```python
from build123d import *

# Parameters (mm, degrees)
CYLINDER959_R           = 1.6
CYLINDER959_DEPTH       = 10
CYLINDER959_PITCH_ANGLE = 90
CYLINDER960_R           = 1.6
CYLINDER960_DEPTH       = 10
CYLINDER960_PITCH_ANGLE = 90
CYLINDER962_R           = 3.1
CYLINDER962_DEPTH       = 2.5
CYLINDER962_PITCH_ANGLE = 90
CYLINDER961_R           = 3.1
CYLINDER961_DEPTH       = 2.5
CYLINDER961_PITCH_ANGLE = 90
BOX562_W                = 41
BOX562_H                = 41
BOX562_DEPTH            = 26
CYLINDER958_R           = 6
CYLINDER958_DEPTH       = 11
CYLINDER958_ROLL_ANGLE  = 90
CYLINDER963_R           = 7
CYLINDER963_DEPTH       = 5
CYLINDER963_ROLL_ANGLE  = 90
BOX563_W                = 10
BOX563_H                = 10
BOX563_DEPTH            = 17
CYLINDER953_R           = 1.2
CYLINDER953_DEPTH       = 10
CYLINDER953_ROLL_ANGLE  = 90
CYLINDER952_R           = 1.2
CYLINDER952_DEPTH       = 10
CYLINDER952_ROLL_ANGLE  = 90
CYLINDER957_R           = 1.25
CYLINDER957_DEPTH       = 15
CYLINDER957_PITCH_ANGLE = 90
CYLINDER955_R           = 1.25
CYLINDER955_DEPTH       = 11
CYLINDER955_PITCH_ANGLE = 90
CYLINDER956_R           = 1.25
CYLINDER956_DEPTH       = 15
CYLINDER956_PITCH_ANGLE = 90
CYLINDER954_R           = 1.25
CYLINDER954_DEPTH       = 11
CYLINDER954_PITCH_ANGLE = 90
BOX561_W                = 10
BOX561_H                = 63
BOX561_DEPTH            = 25.5
FILLET358_R             = 3
BOX560_W                = 16
BOX560_H                = 60
BOX560_DEPTH            = 17
FILLET359_R             = 3


with BuildPart() as cylinder1122:
    # Cylinder959 → Cylinder959 (new body)
    with BuildSketch(Plane.XY):
        Circle(CYLINDER959_R)
    extrude(amount=CYLINDER959_DEPTH)


with BuildPart() as cylinder1122_1:
    # Cylinder959 pitch: moved
    add(cylinder1122.part.rotate(Axis((0, 0, 0), (0, 1, 0)), CYLINDER959_PITCH_ANGLE))


with BuildPart() as cylinder1122_2:
    # Cylinder959 placement: moved
    add(cylinder1122_1.part.moved(Location((13.5, 83, -11))))


with BuildPart() as cylinder1123:
    # Cylinder960 → Cylinder960 (new body)
    with BuildSketch(Plane.XY):
        Circle(CYLINDER960_R)
    extrude(amount=CYLINDER960_DEPTH)


with BuildPart() as cylinder1123_1:
    # Cylinder960 pitch: moved
    add(cylinder1123.part.rotate(Axis((0, 0, 0), (0, 1, 0)), CYLINDER960_PITCH_ANGLE))


with BuildPart() as cylinder1123_2:
    # Cylinder960 placement: moved
    add(cylinder1123_1.part.moved(Location((13.5, 91, -11))))


with BuildPart() as cylinder1125:
    # Cylinder962 → Cylinder962 (new body)
    with BuildSketch(Plane.XY):
        Circle(CYLINDER962_R)
    extrude(amount=CYLINDER962_DEPTH)


with BuildPart() as cylinder1125_1:
    # Cylinder962 pitch: moved
    add(cylinder1125.part.rotate(Axis((0, 0, 0), (0, 1, 0)), CYLINDER962_PITCH_ANGLE))


with BuildPart() as cylinder1125_2:
    # Cylinder962 placement: moved
    add(cylinder1125_1.part.moved(Location((13.5, 83, -11))))


with BuildPart() as fusion603:
    # Cylinder961 → Cylinder961 (new body)
    with BuildSketch(Plane.XY):
        Circle(CYLINDER961_R)
    extrude(amount=CYLINDER961_DEPTH)


with BuildPart() as fusion603_1:
    # Cylinder961 pitch: moved
    add(fusion603.part.rotate(Axis((0, 0, 0), (0, 1, 0)), CYLINDER961_PITCH_ANGLE))


with BuildPart() as fusion603_2:
    # Cylinder961 placement: moved
    add(fusion603_1.part.moved(Location((13.5, 91, -11))))

    # Fusion603: union Cylinder1122, Cylinder1123, Cylinder1125
    add(cylinder1122_2.part)
    add(cylinder1123_2.part)
    add(cylinder1125_2.part)


with BuildPart() as cube753:
    # Box562 → Box562 (new body)
    with BuildSketch(Plane(origin=(19.5, 64.5, -21.5), x_dir=(1, 0, 0), z_dir=(0, 0, 1))):
        with Locations((20.5, 20.5)):
            Rectangle(BOX562_W, BOX562_H)
    extrude(amount=BOX562_DEPTH)


with BuildPart() as cylinder1121:
    # Cylinder958 → Cylinder958 (new body)
    with BuildSketch(Plane.XY):
        Circle(CYLINDER958_R)
    extrude(amount=CYLINDER958_DEPTH)


with BuildPart() as cylinder1121_1:
    # Cylinder958 roll: moved
    add(cylinder1121.part.rotate(Axis((0, 0, 0), (1, 0, 0)), CYLINDER958_ROLL_ANGLE))


with BuildPart() as cylinder1121_2:
    # Cylinder958 placement: moved
    add(cylinder1121_1.part.moved(Location((37, 64.5, -11))))


with BuildPart() as cylinder1126:
    # Cylinder963 → Cylinder963 (new body)
    with BuildSketch(Plane.XY):
        Circle(CYLINDER963_R)
    extrude(amount=CYLINDER963_DEPTH)


with BuildPart() as cylinder1126_1:
    # Cylinder963 roll: moved
    add(cylinder1126.part.rotate(Axis((0, 0, 0), (1, 0, 0)), CYLINDER963_ROLL_ANGLE))


with BuildPart() as cylinder1126_2:
    # Cylinder963 placement: moved
    add(cylinder1126_1.part.moved(Location((37, 64.5, -11))))


with BuildPart() as fusion604:
    # Box563 → Box563 (new body)
    with BuildSketch(Plane(origin=(37, 55, -19.5), x_dir=(1, 0, 0), z_dir=(0, 0, 1))):
        with Locations((5, 5)):
            Rectangle(BOX563_W, BOX563_H)
    extrude(amount=BOX563_DEPTH)

    # Fusion604: union Cube753, Cylinder1121, Cylinder1126
    add(cube753.part)
    add(cylinder1121_2.part)
    add(cylinder1126_2.part)


with BuildPart() as cylinder1116:
    # Cylinder953 → Cylinder953 (new body)
    with BuildSketch(Plane.XY):
        Circle(CYLINDER953_R)
    extrude(amount=CYLINDER953_DEPTH)


with BuildPart() as cylinder1116_1:
    # Cylinder953 roll: moved
    add(cylinder1116.part.rotate(Axis((0, 0, 0), (1, 0, 0)), CYLINDER953_ROLL_ANGLE))


with BuildPart() as cylinder1116_2:
    # Cylinder953 placement: moved
    add(cylinder1116_1.part.moved(Location((3, 10, 10))))


with BuildPart() as fusion600:
    # Cylinder952 → Cylinder952 (new body)
    with BuildSketch(Plane.XY):
        Circle(CYLINDER952_R)
    extrude(amount=CYLINDER952_DEPTH)


with BuildPart() as fusion600_1:
    # Cylinder952 roll: moved
    add(fusion600.part.rotate(Axis((0, 0, 0), (1, 0, 0)), CYLINDER952_ROLL_ANGLE))


with BuildPart() as fusion600_2:
    # Cylinder952 placement: moved
    add(fusion600_1.part.moved(Location((3, 60, 10))))

    # Fusion600: union Cylinder1116
    add(cylinder1116_2.part)


with BuildPart() as fusion600_3:
    # Fusion600 placement: moved
    add(fusion600_2.part.moved(Location((0, 0, 2))))


with BuildPart() as cylinder1120:
    # Cylinder957 → Cylinder957 (new body)
    with BuildSketch(Plane.XY):
        Circle(CYLINDER957_R)
    extrude(amount=CYLINDER957_DEPTH)


with BuildPart() as cylinder1120_1:
    # Cylinder957 pitch: moved
    add(cylinder1120.part.rotate(Axis((0, 0, 0), (0, 1, 0)), CYLINDER957_PITCH_ANGLE))


with BuildPart() as cylinder1120_2:
    # Cylinder957 placement: moved
    add(cylinder1120_1.part.moved(Location((-2, 23, 20))))


with BuildPart() as cylinder1118:
    # Cylinder955 → Cylinder955 (new body)
    with BuildSketch(Plane.XY):
        Circle(CYLINDER955_R)
    extrude(amount=CYLINDER955_DEPTH)


with BuildPart() as cylinder1118_1:
    # Cylinder955 pitch: moved
    add(cylinder1118.part.rotate(Axis((0, 0, 0), (0, 1, 0)), CYLINDER955_PITCH_ANGLE))


with BuildPart() as cylinder1118_2:
    # Cylinder955 placement: moved
    add(cylinder1118_1.part.moved(Location((-2, 13.5, 4))))


with BuildPart() as cylinder1119:
    # Cylinder956 → Cylinder956 (new body)
    with BuildSketch(Plane.XY):
        Circle(CYLINDER956_R)
    extrude(amount=CYLINDER956_DEPTH)


with BuildPart() as cylinder1119_1:
    # Cylinder956 pitch: moved
    add(cylinder1119.part.rotate(Axis((0, 0, 0), (0, 1, 0)), CYLINDER956_PITCH_ANGLE))


with BuildPart() as cylinder1119_2:
    # Cylinder956 placement: moved
    add(cylinder1119_1.part.moved(Location((-2, 57, 20))))


with BuildPart() as fusion601:
    # Cylinder954 → Cylinder954 (new body)
    with BuildSketch(Plane.XY):
        Circle(CYLINDER954_R)
    extrude(amount=CYLINDER954_DEPTH)


with BuildPart() as fusion601_1:
    # Cylinder954 pitch: moved
    add(fusion601.part.rotate(Axis((0, 0, 0), (0, 1, 0)), CYLINDER954_PITCH_ANGLE))


with BuildPart() as fusion601_2:
    # Cylinder954 placement: moved
    add(fusion601_1.part.moved(Location((-2, 66.5, 4))))

    # Fusion599: union Cylinder1120, Cylinder1118, Cylinder1119
    add(cylinder1120_2.part)
    add(cylinder1118_2.part)
    add(cylinder1119_2.part)


with BuildPart() as fusion601_3:
    # Fusion599 placement: moved
    add(fusion601_2.part.moved(Location((-10, -10, 1))))

    # Fusion601: union Fusion600
    add(fusion600_3.part)


with BuildPart() as fusion601_4:
    # Fusion601 placement: moved
    add(fusion601_3.part.moved(Location((25.5, 55, -23))))


with BuildPart() as fillet358:
    # Box561 → Box561 (new body)
    with BuildSketch(Plane(origin=(-12, 0, -5), x_dir=(1, 0, 0), z_dir=(0, 0, 1))):
        with Locations((5, 31.5)):
            Rectangle(BOX561_W, BOX561_H)
    extrude(amount=BOX561_DEPTH)

    # Fillet358
    fillet358_edges = [fillet358.edges().sort_by_distance(p)[0] for p in [
        (-7, 0, -5),
        (-7, 0, 20.5),
        (-7, 63, -5),
        (-7, 63, 20.5),
    ]]
    fillet(fillet358_edges, radius=FILLET358_R)


with BuildPart() as fillet358_1:
    # Fillet358 placement: moved
    add(fillet358.part.moved(Location((25.5, 53.5, -16.5))))


with BuildPart() as cross_member_front_lifted:
    # Box560 → Box560 (new body)
    with BuildSketch(Plane(origin=(-2, 0, 1.5), x_dir=(1, 0, 0), z_dir=(0, 0, 1))):
        with Locations((8, 30)):
            Rectangle(BOX560_W, BOX560_H)
    extrude(amount=BOX560_DEPTH)

    # Fillet359
    fillet359_edges = [cross_member_front_lifted.edges().sort_by_distance(p)[0] for p in [
        (6, 0, 1.5),
        (6, 0, 18.5),
        (6, 60, 1.5),
        (6, 60, 18.5),
    ]]
    fillet(fillet359_edges, radius=FILLET359_R)


with BuildPart() as cross_member_front_lifted_1:
    # Fillet359 placement: moved
    add(cross_member_front_lifted.part.moved(Location((25.5, 55, -21))))

    # Fusion605: union Fillet358
    add(fillet358_1.part)

    # Cut698: cut Fusion601
    add(fusion601_4.part, mode=Mode.SUBTRACT)

    # Cut699: cut Fusion604
    add(fusion604.part, mode=Mode.SUBTRACT)

    # Cut700: cut Fusion603
    add(fusion603_2.part, mode=Mode.SUBTRACT)


solid = cross_member_front_lifted_1.part
```
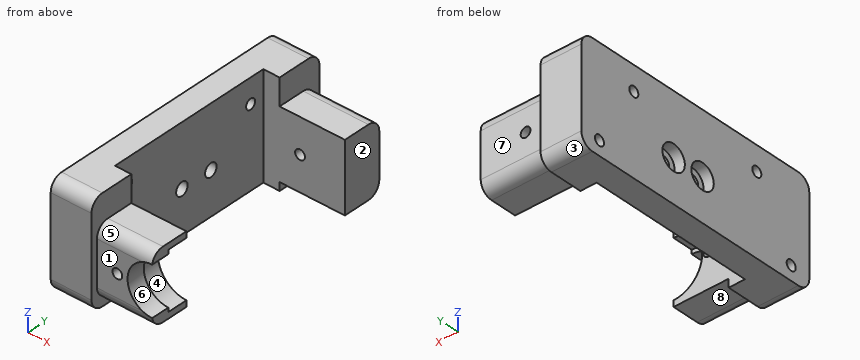
Could you check a few things on this model? Use its own coordinates, in mm. Face numbers are marked on the shaded views. A direction names the side the tool comes from. Coordinates: 2 decimals unless noted, no trailing zeros. Loops run counter-clockwise (first coordinate to the right, second up) from the corner with the lowest first, then second, coordinate; pieces in that order, holes last.
1) Please list where these lines run through material, in increasing order: line 1 along Y through (x, z) = (17, -18); line 2 along Y through (x, z) = (14.25, -11); line 3 along Y through (x, z) = (22, -18).
Reported:
line 1: y = 53.5 to 57.25, 59.75 to 110.25, 112.75 to 116.5
line 2: y = 53.5 to 79.9, 86.1 to 87.9, 94.1 to 116.5
line 3: y = 53.5 to 57.25, 59.75 to 64.5, 105.5 to 110.25, 112.75 to 116.5
2) Imagine slicing it at D-D (y = 83). List the corners of the cut face in (x, z) for me.
Reported:
outline: (13.5, -21.5) - (19.5, -21.5) - (19.5, -12.6) - (16, -12.6) - (16, -14.1) - (13.5, -14.1) - close; (13.5, -7.9) - (16, -7.9) - (16, -9.4) - (19.5, -9.4) - (19.5, 4) - (13.5, 4) - close
3) Thinking about a two-plate mould opening in Y: for the marked faces 1, 2, 3 and 4, which applies, released by +Y, released by -Y, zero draft, split by the parting line, or undercut?
Reported:
face 1: released by -Y
face 2: zero draft
face 3: released by +Y
face 4: undercut
4) Imagine slicing it at B-B (x = 26.5). List the corners of the cut face in (y, z) for me, and give its area (3 significant figures).
Reported:
outline: (55, -16.5) arc R3 ccw to (58, -19.5) - (64.5, -19.5) - (64.5, -2.5) - (58, -2.5) arc R3 ccw to (55, -5.5) - close; (105.5, -19.5) - (112, -19.5) arc R3 ccw to (115, -16.5) - (115, -5.5) arc R3 ccw to (112, -2.5) - (105.5, -2.5) - close
area: 315 mm2
5) Will these pins go through, and if not, where does the flat tip stop? pin 1 Ø3 at (y, z) = (111, -18.5) entering from -X; pin 2 Ø2 at (y, z) = (58.5, -18) entering from -X; pin 3 Ø3 at (y, z) = (92, -11.5) entering from -X; pin 4 Ø1.9 at (x, z) = (28.5, -11) entering from -Y.
Reported:
pin 1: stops at x = 13.5
pin 2: stops at x = 24.5
pin 3: stops at x = 16
pin 4: passes through
6) Which directions (+Z, -Z, +X, -X, +Y, -Y) give clear straight access to the entire face, cutting with the end or side of a thin tool? Please do the marked faces 5, 6, 7 and 8.
Reported:
face 5: +Z, +X, -Y
face 6: +X, -Y
face 7: +Z, -Z, +X, +Y
face 8: -Z, +X, +Y, -Y
7) Imagine slicing it at A-A (y = 68). List the corners of the cut face in (x, z) for me, and give its area (3 significant figures).
Reported:
outline: (13.5, -21.5) - (19.5, -21.5) - (19.5, -3.25) - (13.5, -3.25) - close; (13.5, -0.75) - (19.5, -0.75) - (19.5, 4) - (13.5, 4) - close
area: 138 mm2
8) Imagine slicing it at C-C (y = 108). List the corners of the cut face in (x, z) for me, and give its area (3 significant figures).
Reported:
outline: (13.5, -21.5) - (23.5, -21.5) - (23.5, -19.5) - (39.5, -19.5) - (39.5, -2.5) - (23.5, -2.5) - (23.5, 4) - (13.5, 4) - close; hole circle Ø2.4 at (28.5, -11)
area: 522 mm2
